The figure shows three views and two pictorial views of one solid part (mm, origin at its lowest corner). Answer the questions. A direction names the side the tool comes from. Coordinates: 2 decimals unless noted, no trailing zeros. Write each loop counter-clockwise with the first axis right and the second up, starting at its lowest first coordinate (ties: lowest second). Pieces come first, ordered by that corner, then holes.
Item 1: Straight lines are drawn through the part: probe 1 along X at (y, z) = (0.25, 20); probe 2 along X at (y, z) = (2.25, 20); probe 3 along Y at (x, z) = (33.5, 16). For each, find the intervals that lie inside material, in ascending order.
Item 2: Section A-A (z = 20) is taken. Give the vertices of the cut face in (x, y).
Item 3: A tool of negligible diameter and unlimited length cuts with its end or side. For the marked faces 1 and 2, from which of +Z, -Z, +X, -X, +Y, -Y can it reach the whole face along a straight path? Write none if from no direction.
Item 4: Section B-B (x = 20) is taken. Give the vertices of the cut face in (y, z).
Item 5: Section C-C (z = 7) is taken. Give the vertices of the cut face in (x, y).
Item 6: Determine the mould class of the marked faces 3, 4 and 5 for opening direction X: released by +X, released by -X, zero draft, split by the parting line, or undercut.
Item 7: Section D-D (x = 33.5) is taken. Give the vertices of the cut face in (y, z), then the cut area to 3 significant figures.
Item 8: Each of these flat-tipped pins is pushed along its axis until it touches: P1, Ø1.5, axis at x = 16.5, y = 6, coming from the -Z side; P2, Ø2, axis at y = 3, z = 15.5, coming from the -X side; P3, Ø5, axis at x = 26.5, y = 2.5, coming from the +Z side. Where does it stop, or does it pass through?
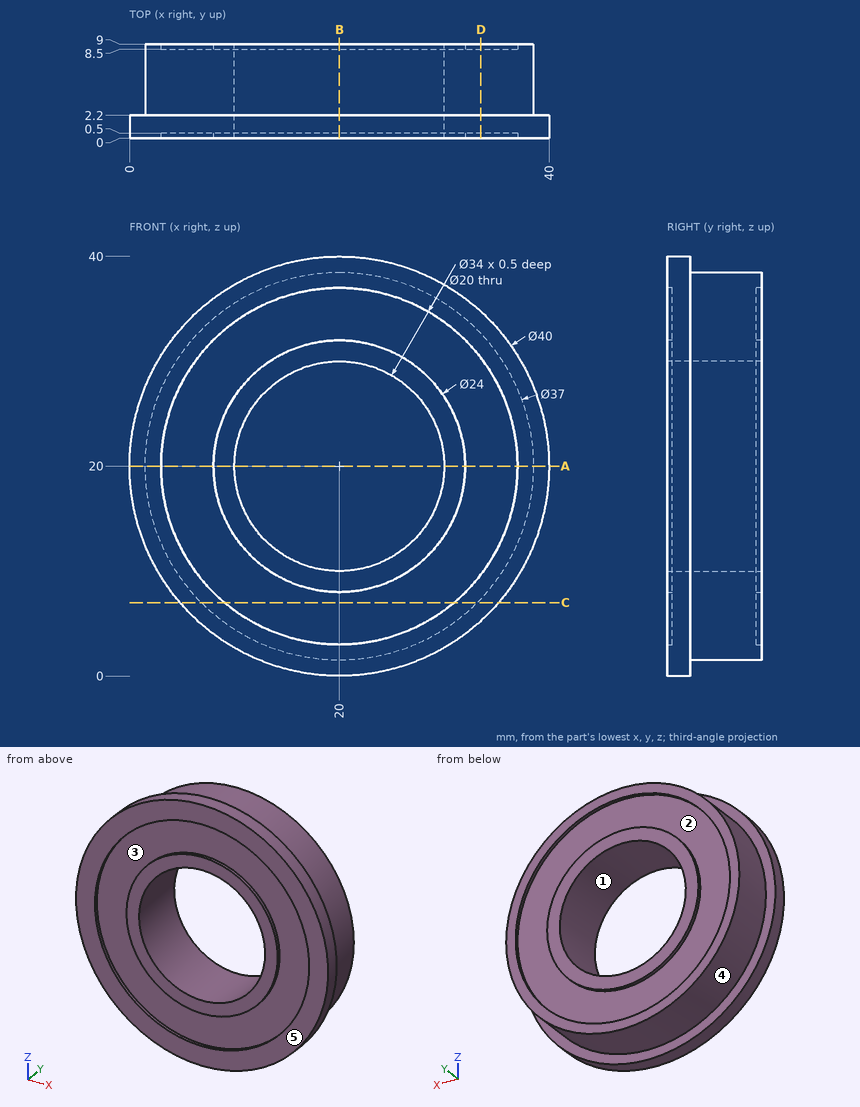
Established:
1. probe 1: x = 0 to 3, 8 to 10, 30 to 32, 37 to 40
1. probe 2: x = 1.5 to 10, 30 to 38.5
1. probe 3: y = 0.5 to 8.5
2. outline: (0, 0) - (3, 0) - (3, 0.5) - (8, 0.5) - (8, 0) - (10, 0) - (10, 9) - (8, 9) - (8, 8.5) - (3, 8.5) - (3, 9) - (1.5, 9) - (1.5, 2.2) - (0, 2.2) - close; (30, 0) - (32, 0) - (32, 0.5) - (37, 0.5) - (37, 0) - (40, 0) - (40, 2.2) - (38.5, 2.2) - (38.5, 9) - (37, 9) - (37, 8.5) - (32, 8.5) - (32, 9) - (30, 9) - close
3. face 1: +Y, -Y
3. face 2: +Y
4. outline: (0, 0) - (2.2, 0) - (2.2, 1.5) - (9, 1.5) - (9, 3) - (8.5, 3) - (8.5, 8) - (9, 8) - (9, 10) - (0, 10) - (0, 8) - (0.5, 8) - (0.5, 3) - (0, 3) - close; (0, 30) - (9, 30) - (9, 32) - (8.5, 32) - (8.5, 37) - (9, 37) - (9, 38.5) - (2.2, 38.5) - (2.2, 40) - (0, 40) - (0, 37) - (0.5, 37) - (0.5, 32) - (0, 32) - close
5. outline: (4.8, 0) - (9.05, 0) - (9.05, 0.5) - (30.95, 0.5) - (30.95, 0) - (35.2, 0) - (35.2, 2.2) - (33.16, 2.2) - (33.16, 9) - (30.95, 9) - (30.95, 8.5) - (9.05, 8.5) - (9.05, 9) - (6.84, 9) - (6.84, 2.2) - (4.8, 2.2) - close
6. face 3: undercut
6. face 4: split by the parting line
6. face 5: zero draft
7. outline: (0, 5.24) - (2.2, 5.24) - (2.2, 7.35) - (9, 7.35) - (9, 9.67) - (8.5, 9.67) - (8.5, 30.33) - (9, 30.33) - (9, 32.65) - (2.2, 32.65) - (2.2, 34.76) - (0, 34.76) - (0, 30.33) - (0.5, 30.33) - (0.5, 9.67) - (0, 9.67) - close
7. area: 216 mm2
8. P1: stops at z = 1.71
8. P2: stops at x = 0.38
8. P3: stops at z = 39.59
